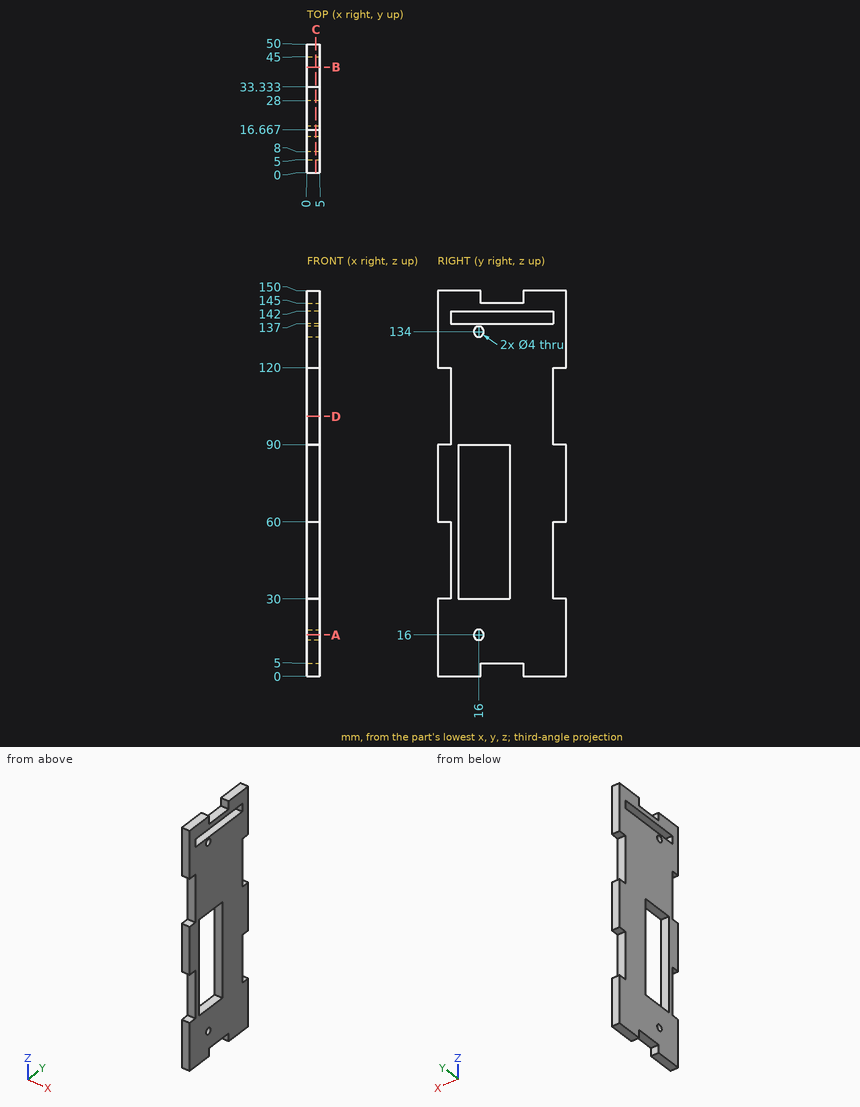
Here's the drawing with two shaded views (mm, measured from the low corner). I have some questions. Coordinates: 2 decimals unless noted, no trailing zeros. Write each loop counter-clockwise with the first axis right and the second up, starting at its lowest first coordinate (ties: lowest second). Pieces come first, ordered by that corner, then holes. Notation, with made-up numbers: M 34.25,13 L 56.25,13 A25 ccw 56.25,44 Z; hole C 18.5,12 d1. An arc over 180 degrees is marked long. Write item = value, one per line. Start each with the question number.
Q1. If I drill on L1, parallel to Z at x = 1.7, y = 20.5; L2, parallel to Y at x = 2.95, z = 134; L3, parallel to Z at x = 0.3, y = 34, over which ranges is the centre line in solid material (lowest first)? Write a range as [from, to].
Q2. If we section it at B-B, the plane y = 41: Write out the boundary of the cut face in (x, z), then the cut area to 3 significant figures.
Q3. If we section it at A-A, the plane z = 16: Write out the boundary of the cut face in (x, y).
Q4. I'm going to push flat-ended pins straight in: pin 1 (2 mm diameter, centred on x = 1, y = 28.5, fed in from -Z); pin 2 (1 mm diameter, centred on x = 2.5, z = 132.5, fed in from -Y). Where does each tip first touch, or does it pass through?
Q5. If we section it at D-D, the plane z = 101: Write out the boundary of the cut face in (x, y), then the cut area to 3 significant figures.
Q6. If we section it at C-C, the plane x = 3.5: State how many separate pieces and enclosed holes the cut face has, then the cut area to 3 significant figures.
Check sheet entries:
q1.L1 = [5, 30], [90, 137], [142, 145]
q1.L2 = [0, 14], [18, 50]
q1.L3 = [0, 137], [142, 150]
q2.outline = M 0,0 L 5,0 L 5,137 L 0,137 Z; M 0,142 L 5,142 L 5,150 L 0,150 Z
q2.area = 725 mm²
q3.outline = M 0,0 L 5,0 L 5,14 L 0,14 Z; M 0,18 L 5,18 L 5,50 L 0,50 Z
q4.pin_1 = 5
q4.pin_2 = 0
q5.outline = M 0,5 L 5,5 L 5,45 L 0,45 Z
q5.area = 200 mm²
q6.separate_pieces = 1
q6.enclosed_holes = 4
q6.area = 5,310 mm²
